Input: part model. Units: mm. Frame: model coordinates. Coordinates: 2 decimals unless noted, no trailing zeros. Order: outer loops, then holes, each group sorted by start corner. A loop starts at its lowest first (then second) coordinate and runs counter-clockwise, first axis right, second up. Notation, with made-up numbers: M 69,-27 L 120,-27 A20 cw 120,-19 Z; hole C 8.5,34 d9. An arc over 180 degrees is marked long. One line per item, written item: value.
Autodesk Inventor part; units mm, degrees
ref_plane "YZ Plane" through (0, 0, 0) normal (1, 0, 0) x (0, 1, 0)
ref_plane "XZ Plane" through (0, 0, 0) normal (0, 1, 0) x (-1, 0, 0)
ref_plane "XY Plane" through (0, 0, 0) normal (0, 0, 1) x (1, 0, 0)
sketch "Sketch1" plane through (0, 0, 0) normal (0, 0, 1) x (1, 0, 0)
  line L0 (0, 0) -> (750, 0)
  line L1 (750, 0) -> (750, 850)
  line L2 (750, 850) -> (0, 850)
  line L3 (0, 850) -> (0, 0)
  dimension "d0" = 750
  dimension "d1" = 850
extrude "Extrusion1" add sketch "Sketch1" along normal blind 40
sketch "Sketch2" plane through (0, 850, 0) normal (0, 1, 0) x (1, 0, 0)
  line L0 (750, 0) -> (0, 0)
  line L1 (0, 0) -> (750, 0)
  line L2 (750, 0) -> (750, -20)
  line L3 (750, -20) -> (0, -20)
  line L4 (0, -20) -> (0, 0)
  dimension "d4" = 750
  dimension "d5" = 20
extrude "Extrusion2" cut sketch "Sketch2" against normal blind 20
sketch "Sketch3" plane through (0, 850, 40) normal (0, 1, 0) x (1, 0, 0)
  line L0 (0, 20) -> (0, 0)
  circle A0 centre (562, 20) radius 5
  circle A1 centre (375, 20) radius 5
  circle A2 centre (188, 20) radius 5
  point P0 (0, 40)
  dimension "d11" = 10
  dimension "d12" = 10
  dimension "d13" = 10
extrude "Extrusion3" cut sketch "Sketch3" against normal blind 40
thread "Thread1"
thread "Thread2"
thread "Thread3"
sketch "Sketch4" plane through (0, 0, 0) normal (0, 0, -1) x (-1, 0, 0)
  line L0 (-750, 720) -> (0, 720)
  line L1 (0, 850) -> (0, 0)
  line L2 (-750, 720) -> (0, 720)
  line L3 (0, 720) -> (0, 690)
  line L4 (0, 690) -> (-750, 690)
  line L5 (-750, 690) -> (-750, 720)
  line L6 (0, 690) -> (-420, 690)
  line L7 (-420, 690) -> (-420, 720)
  line L8 (-420, 720) -> (0, 720)
  line L9 (0, 720) -> (0, 690)
  dimension "d23" = 30
  dimension "d24" = 420
  dimension "d25" = 30
extrude "Extrusion4" cut sketch "Sketch4" against normal blind 20 contours L0 L7 L4 L5
sketch "Sketch5" plane through (0, 0, 0) normal (0, 0, -1) x (-1, 0, 0)
  line L0 (-750, 850) -> (0, 850)
  line L1 (0, 850) -> (-300, 850)
  line L2 (-300, 850) -> (-300, 550)
  line L3 (-300, 550) -> (0, 550)
  line L4 (0, 550) -> (0, 850)
  line L5 (-300, 850) -> (-270, 850)
  line L6 (-270, 850) -> (-270, 550)
  line L7 (-270, 550) -> (-300, 550)
  line L8 (-300, 550) -> (-300, 850)
  point P0 (0, 0)
  dimension "d28" = 300
  dimension "d29" = 300
  dimension "d30" = 30
extrude "Extrusion5" cut sketch "Sketch5" against normal blind 20 contours L0 L6 L3 L2
sketch "Sketch6" plane through (0, 0, 0) normal (0, 0, -1) x (-1, 0, 0)
  circle A0 centre (-600, 705) radius 5
  circle A1 centre (-380, 705) radius 5
  line L0 (-270, 550) -> (-300, 550)
  circle A2 centre (-285, 750) radius 5
  circle A3 centre (-285, 650) radius 5
  point P0 (0, 0)
  point P1 (-750, 690)
  point P2 (-300, 830)
  dimension "d37" = 10
  dimension "d38" = 10
  dimension "d44" = 10
  dimension "d45" = 10
extrude "Extrusion6" cut sketch "Sketch6" against normal blind 81.4375
thread "Thread4"
thread "Thread5"
thread "Thread6"
thread "Thread7"
properties part number "wall"
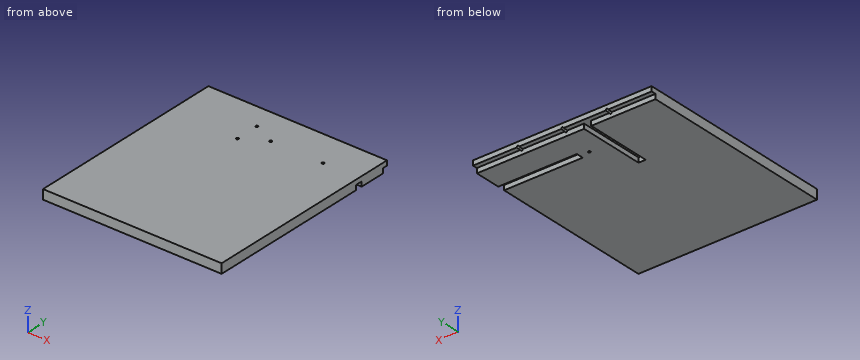
(1) Ray query, line 1 (Y direction, x = 285, z = 33.5); line 2 (Y direction, x = 600, z = 30.75); line 3 (Z direction, x = 188, y = 824). Return the intervals inside material, ascending. Write a range as from..to.
Data:
line 1: y = 0..645, 655..745, 755..850
line 2: y = 0..700, 710..850
line 3: z = 0..15, 25..40
(2) Cut plane B-B on x = 540.5. Output: boundary loops of the cut face in (y, z).
Data:
outline: M 0,0 L 690,0 L 690,20 L 720,20 L 720,0 L 830,0 L 830,20 L 850,20 L 850,40 L 0,40 Z
(3) Cut plane A-A on z = 9. Output: boundary loops of the cut face in (x, y), plus the area to 3 significant figures.
Data:
outline: M 0,0 L 750,0 L 750,690 L 420,690 L 420,720 L 750,720 L 750,830 L 300,830 L 300,550 L 270,550 L 270,830 L 0,830 Z; hole C 380,705 d10
area: 604,000 mm2
(4) First-contact query: pin 1 (16 mm diameter, centred on x = 600, y = 705, fed in from -Z); pin 2 (22 mm diameter, centred on x = 413.5, z = 5, fed in from +Y); pin 3 (10 mm diameter, centred on y = 707.5, z = 7.5, fed in from +X). Flat tips, straight axial feed; report the tip coordinate or a pass-through.
Data:
pin 1: stops at z = 20
pin 2: stops at y = 830
pin 3: stops at x = 420
